Part model, mm, in its own coordinate system. Give positions to 0.01 mm unless a question says otherwise; leave off trailing zeros. Order: outer loops, then holes, each group sorted by start corner. A loop starts at its lowest first (then second) coordinate and runs counter-clockwise, first axis right, second up. Notation, with made-up numbers: M -1,-9.5 L 47,-9.5 A12 cw 47,9.5 Z; hole C -9.75,67 d9. An arc over 180 degrees is marked long. Return JSON: item names as keys, results as strings.
from build123d import *

# Parameters (mm, degrees)
SKETCH1_R           = 75
BOSS_EXTRUDE1_DEPTH = 100
BOSS_EXTRUDE1_TAPER = 12
SKETCH3_R           = 70
CUT_EXTRUDE1_DEPTH  = 80
CUT_EXTRUDE1_TAPER  = 12
FILLET1_R           = 10
SKETCH4_R           = 15
CUT_EXTRUDE2_DEPTH  = 90
SKETCH5_R           = 14.5
SKETCH5_R_2         = 12.5
BOSS_EXTRUDE2_DEPTH = 30
SKETCH6_R           = 12.5
CUT_EXTRUDE3_DEPTH  = 30
SKETCH7_R           = 73.5
CUT_EXTRUDE4_DEPTH  = 130


with BuildPart() as part:
    # Sketch1 → Boss-Extrude1 (new body)
    with BuildSketch(Plane(origin=(0, 0, 0), x_dir=(1, 0, 0), z_dir=(0, 1, 0))):
        Circle(SKETCH1_R)
    extrude(amount=-BOSS_EXTRUDE1_DEPTH, taper=BOSS_EXTRUDE1_TAPER)

    # Sketch3 → Cut-Extrude1 (cut)
    with BuildSketch(Plane(origin=(0, -10, 0), x_dir=(1, 0, 0), z_dir=(0, 1, 0))):
        Circle(SKETCH3_R)
    extrude(amount=-CUT_EXTRUDE1_DEPTH, taper=CUT_EXTRUDE1_TAPER, mode=Mode.SUBTRACT)

    # Fillet1
    fillet1_edges = [part.edges().sort_by_distance(p)[0] for p in [
        (-75, 0, 0),
    ]]
    fillet(fillet1_edges, radius=FILLET1_R)

    # Sketch4 → Cut-Extrude2 (cut)
    with BuildSketch(Plane.XY):
        with Locations((-25, -40)):
            Circle(SKETCH4_R)
        with Locations((25, -40)):
            Circle(SKETCH4_R)
        with BuildLine():
            Line((-15, -70), (15, -70))
            ThreePointArc((15, -70), (0, -85), (-15, -70))
        make_face()
    extrude(amount=-CUT_EXTRUDE2_DEPTH, mode=Mode.SUBTRACT)

    # Sketch5 → Boss-Extrude2 (add)
    with BuildSketch(Plane.XZ.offset(100)):
        Circle(SKETCH5_R)
        Circle(SKETCH5_R_2, mode=Mode.SUBTRACT)
    extrude(amount=BOSS_EXTRUDE2_DEPTH)

    # Sketch6 → Cut-Extrude3 (cut)
    with BuildSketch(Plane.XZ.offset(100)):
        Circle(SKETCH6_R)
    extrude(amount=-CUT_EXTRUDE3_DEPTH, mode=Mode.SUBTRACT)

    # Sketch7 → Cut-Extrude4 (cut)
    with BuildSketch(Plane(origin=(0, -12.079116908, 0), x_dir=(1, 0, 0), z_dir=(0, 1, 0))):
        Circle(SKETCH7_R)
    extrude(amount=-CUT_EXTRUDE4_DEPTH, mode=Mode.SUBTRACT)


solid = part.part
Q1. Band-saw the part on A-A (x = 0). Give the cut face in (y, z), then the cut area to 3 significant figures.
Established:
{"outline": "M -12.08,-72.43 A10 ccw 0,-62.65 L 0,62.65 A10 ccw -12.08,72.43 L -12.08,69.56 L -10,70 L -10,-70 L -12.08,-69.56 Z", "area": "1,420 mm²"}
Q2. Pin check, flat tips, straight feed: pin 1 (1 mm diameter, centred on y = -3, z = 0, fed in from -X); pin 2 (3 mm diameter, centred on y = -10, z = -5.5, fed in from +X); pin 3 (5 mm diameter, centred on x = 25, y = -8, fed in from +Z). Stop position of each tip, or through.
Established:
{"pin 1": "stops at x = -70.25", "pin 2": "stops at x = 72.54", "pin 3": "stops at z = 68.96"}
Q3. Probe line 1 along Y through (x, z) = (30, -45); line 2 along Z through (x, y) = (-53, -11.25); line 3 along Z through (x, y) = (-50, -11.25). List the from-to ranges inside material, lowest first.
Established:
{"line 1": "y = -10 to 0", "line 2": "z = -49.58 to -45.32, 45.32 to 49.58", "line 3": "z = -52.6 to -48.61, 48.61 to 52.6"}
Q4. Two-plate mould, pull along X, no slides. Class faces 1 (the flat face through (-1, 0, -1)), 2 (the flat face through (-1, -10, -1)): +X half, -X half, draft (parallel to the pull), parting line (faces both ways), or undercut.
Established:
{"face 1": "draft", "face 2": "undercut"}
Q5. Band-saw the part on B-B (y = -4). Give the cut face in (x, z), then the cut area to 3 significant figures.
Established:
{"outline": "C 0,0 d141.3", "area": "15,700 mm²"}
